The listing builds one solid part. Answer for the finished solid, in the listing's coordinates (mm). A direction names the side the tool comes from. Give positions to 0.01 mm unless a question says otherwise; leave off trailing zeros. Write each loop counter-clockwise with the first axis right and the second up, starting at its lowest first coordinate (ties: lowest second). Pieces come first, ordered by that corner, then holes. Notation, with made-up numbers: (89.25, 76) - (113.25, 76) arc R13 ccw to (113.25, 101) - close; hole circle Ø5 at (25, 7). An arc over 180 degrees is marked (long way). Answer as CSV lines item,"result". Start each with the question number.
(1) Find section D-D (x = -20.5). Write down the section's boundary in (y, z).
(2) Find section B-B (x = -31.5). Write down the section's boundary in (y, z).
(3) For a pull along Z with two mould halves and no side action, classify faces 1 (the face through (-25, -12, -10)), 2 (the face through (-28, -11, -10)), 3 (the face through (-38.059, -12.735, -1.391)) as pulls with the +Z half, pulls with the -Z half, needs draft (parallel to the pull), parting line crosses it, or undercut.
(4) Straight lines are drawn through the part: probe 1 along X at (y, z) = (-10, -13.5); probe 2 along Z at (x, y) = (-26.5, -8); probe 3 along X at (y, z) = (-13.5, -6.75). For each, find the intervals that lie inside material, in ascending order.
(5) Find section C-C (x = 0). Write down the section's boundary in (y, z).
(6) Each of these flat-tipped pins is pushed along its axis until it touches: pin 1 Ø0.9 at (x, z) = (-16.5, 1) entering from -Y; pin 2 Ø5.5 at (x, y) = (0, 0) entering from -Z; pin 3 Ø2 at (x, z) = (-26.5, -10) entering from +Y; pin 4 Ø3 at (y, z) = (-4, -17.5) entering from -X. Where does it stop, or does it pass through?
(7) Find section A-A (y = 0). Write down the section's boundary in (x, z), then the cut area to 3 significant figures.
(8) For faces 4 (the face through (-37.832, -11.752, -19.495)), 5 (the face through (-38.126, -12.665, -6.773)), 6 (the face through (-26, -8.4, -8)), determine the directions among +Z, -Z, +X, -X, +Y, -Y from which every point of the face is accessible in a straight line to the end or side of a thin tool.
from build123d import *

# Parameters (mm, degrees)
SKETCH1_R           = 1.7
BOSS_EXTRUDE1_DEPTH = 3
BOSS_EXTRUDE2_DEPTH = 3
BOSS_EXTRUDE3_DEPTH = 20
BOSS_EXTRUDE4_DEPTH = 3
FILLET1_R           = 3
BOSS_EXTRUDE5_REACH = 38.788
BOSS_EXTRUDE6_DEPTH = 3
BOSS_EXTRUDE7_DEPTH = 3
FILLET3_R           = 1


with BuildPart() as part:
    # Sketch1 → Boss-Extrude1 (new body)
    with BuildSketch(Plane.XY):
        with BuildLine():
            Line((-3.774917218, 2.8), (-48, 2.8))
            Line((-48, 2.8), (-48, -10.2))
            Line((-48, -10.2), (-28, -10.2))
            Line((-28, -10.2), (-28, -8.4))
            Line((-28, -8.4), (-10.549988409, -8.4))
            Line((-10.549988409, -8.4), (1.462547038, -4.466649321))
            ThreePointArc((1.462547038, -4.466649321), (3.812848286, 2.748124442), (-3.774917218, 2.8))
        make_face()
        Circle(SKETCH1_R, mode=Mode.SUBTRACT)
    extrude(amount=BOSS_EXTRUDE1_DEPTH)

    # Sketch2 → Boss-Extrude2 (add)
    with BuildSketch(Plane.ZY.offset(48)):
        Polygon((-15.5, 2.8), (3, 2.8), (3, -10.2), (-5.660254038, -15.2), (-15.5, -15.2), align=None)
    extrude(amount=BOSS_EXTRUDE2_DEPTH)

    # Sketch3 → Boss-Extrude3 (add)
    with BuildSketch(Plane(origin=(-48, 0, 0), x_dir=(0, 0, -1), z_dir=(1, 0, 0))):
        Polygon((-3, -10.2), (0, -10.2), (13.737387097, -15.2), (5.660254038, -15.2), align=None)
    extrude(amount=BOSS_EXTRUDE3_DEPTH)

    # Sketch4 → Boss-Extrude4 (add)
    with BuildSketch(Plane(origin=(-28, 0, 0), x_dir=(0, 0, -1), z_dir=(1, 0, 0))):
        Polygon((-3, -10.2), (-3, -8.4), (15.5, -8.4), (15.5, -15.2), (5.660254038, -15.2), align=None)
    extrude(amount=BOSS_EXTRUDE4_DEPTH)

    # Fillet1
    fillet1_edges = [part.edges().sort_by_distance(p)[0] for p in [
        (-10.549988409, -8.4, 1.5),
        (-25, -8.4, 1.5),
        (-3.774917218, 2.8, 1.5),
    ]]
    fillet(fillet1_edges, radius=FILLET1_R)

    # Boss-Extrude5: up to this face of the body (flat: up to its plane)
    boss_extrude5_end = Plane(part.part.faces().sort_by_distance((-51, -5.690054126, -6.692488054))[0])
    # Sketch6 → Boss-Extrude5 (add, up to the picked face)
    with BuildSketch(Plane(origin=(-25, 0, 0), x_dir=(0, 0, -1), z_dir=(1, 0, 0)), mode=Mode.PRIVATE) as boss_extrude5_sk1:
        Polygon((15.5, -8.4), (23.60392443, -15.2), (21.60392443, -15.2), (15.5, -10.078199262), align=None)
    boss_extrude5_tool1 = split(extrude(boss_extrude5_sk1.sketch, amount=-BOSS_EXTRUDE5_REACH, mode=Mode.PRIVATE), bisect_by=boss_extrude5_end, keep=Keep.BOTH, mode=Mode.PRIVATE)
    add(boss_extrude5_tool1.solids().sort_by(Axis((-25, -12.199864, -19.075423), (-1, 0, 0)))[0])

    # Sketch7 → Boss-Extrude6 (add)
    with BuildSketch(Plane(origin=(-25, 0, 0), x_dir=(0, 0, -1), z_dir=(1, 0, 0))):
        Polygon((15.5, -15.2), (21.60392443, -15.2), (15.5, -10.078199262), align=None)
    extrude(amount=-BOSS_EXTRUDE6_DEPTH)

    # Sketch8 → Boss-Extrude7 (add)
    with BuildSketch(Plane.ZY.offset(51)):
        Polygon((-21.60392443, -15.2), (-15.5, -10.078199262), (-15.5, -15.2), align=None)
    extrude(amount=-BOSS_EXTRUDE7_DEPTH)

    # Fillet3
    fillet3_edges = [part.edges().sort_by_distance(p)[0] for p in [
        (-25, -11.8, -19.551962215),
        (-51, -11.8, -19.551962215),
        (-28, -12.639099631, -18.551962215),
        (-48, -12.639099631, -18.551962215),
        (-28, -12.7, -6.868693549),
        (-48, -12.7, -6.868693549),
        (-25, -9.9, 0),
    ]]
    fillet(fillet3_edges, radius=FILLET3_R)


solid = part.part
Result set:
1,outline,"(-8.4, 0) - (2.8, 0) - (2.8, 3) - (-8.4, 3) - close"
2,outline,"(-15.2, -23.6) - (-8.4, -15.5) - (-10.08, -15.5) - (-15.2, -21.6) - close; (-15.2, -13.74) - (-10.2, 0) - (2.8, 0) - (2.8, 3) - (-10.2, 3) - (-15.2, -5.66) - close"
3,face 1,"needs draft"
3,face 2,"undercut"
3,face 3,"pulls with the +Z half"
4,probe 1,"-51 to -48, -28 to -25"
4,probe 2,"0 to 3"
4,probe 3,"-51 to -25"
5,outline,"(-4.95, 0) - (-1.7, 0) - (-1.7, 3) - (-4.95, 3) - close; (1.7, 0) - (4.7, 0) - (4.7, 3) - (1.7, 3) - close"
6,pin 1,"y = -8.4"
6,pin 2,"z = 0"
6,pin 3,"y = -8.4"
6,pin 4,"through"
7,outline,"(-51, -15.5) - (-48, -15.5) - (-48, 0) - (-1.7, 0) - (-1.7, 3) - (-51, 3) - close; (1.7, 0) - (4.7, 0) - (4.7, 3) - (1.7, 3) - close"
7,area,"203 mm^2"
8,face 4,"-Z, +X, -X, +Y"
8,face 5,"+Y"
8,face 6,"-Z, +X, +Y"
